Autodesk Inventor part; units mm, degrees
ref_plane "YZ Plane" through (0, 0, 0) normal (1, 0, 0) x (0, 1, 0)
ref_plane "XZ Plane" through (0, 0, 0) normal (0, 1, 0) x (-1, 0, 0)
ref_plane "XY Plane" through (0, 0, 0) normal (0, 0, 1) x (1, 0, 0)
sketch "Sketch1" plane through (0, 0, 0) normal (0, 0, 1) x (1, 0, 0)
  line L0 (0, 0) -> (-38.1, 0)
  line L1 (0, 0) -> (0, 114.3)
  line L2 (0, 114.3) -> (-38.1, 114.3)
  line L3 (-38.1, 114.3) -> (-38.1, 0)
  line L4 (-38.1, 114.3) -> (-31.75, 114.3)
  line L5 (-31.75, 114.3) -> (-31.75, 12.7)
  line L6 (0, 114.3) -> (-6.35, 114.3)
  line L7 (-6.35, 114.3) -> (-6.35, 12.7)
  circle A0 centre (-31.75, 12.7) radius 2.1463
  circle A1 centre (-6.35, 12.7) radius 2.1463
  dimension "d0" = 38.1
  dimension "d1" = 114.3
  dimension "d2" = 6.35
  dimension "d3" = 101.6
  dimension "d4" = 6.35
  dimension "d5" = 4.2926
  dimension "d6" = 4.2926
  dimension "d7" = 101.6
extrude "Plate1" add sketch "Sketch1" along normal blind 3.175
sketch "Sketch3" plane through (0, 0, 3.175) normal (0, 0, 1) x (1, 0, 0)
  line L0 (0, 114.3) -> (0, 0)
  line L1 (-38.1, 114.3) -> (0, 114.3)
  line L2 (-38.1, 0) -> (-38.1, 114.3)
  line L3 (-38.1, 114.3) -> (-38.1, 107.95)
  line L4 (-38.1, 107.95) -> (-31.75, 107.95)
  circle A0 centre (-31.75, 107.95) radius 3.3782
  line L5 (0, 114.3) -> (0, 107.95)
  line L6 (0, 107.95) -> (-6.35, 107.95)
  circle A1 centre (-6.35, 107.95) radius 3.3782
  line L7 (-38.1, 107.95) -> (-38.1, 57.15)
  line L8 (-38.1, 57.15) -> (-31.75, 57.15)
  line L9 (0, 57.15) -> (-6.35, 57.15)
  circle A2 centre (-31.75, 57.15) radius 3.3782
  circle A3 centre (-6.35, 57.15) radius 3.3782
  line L10 (-38.1, 114.3) -> (-38.1, 82.55)
  line L11 (-38.1, 82.55) -> (-19.05, 82.55)
  circle A4 centre (-19.05, 82.55) radius 14.2875
  dimension "d19" = 6.35
  dimension "d20" = 6.35
  dimension "d21" = 6.7564
  dimension "d22" = 6.35
  dimension "d23" = 6.35
  dimension "d24" = 6.7564
  dimension "d25" = 50.8
  dimension "d26" = 6.35
  dimension "d27" = 6.35
  dimension "d28" = 57.15
  dimension "d29" = 6.7564
  dimension "d30" = 6.7564
  dimension "d31" = 31.75
  dimension "d32" = 28.575
extrude "Cut1" cut sketch "Sketch3" against normal blind 3.175
equation "\"d33\" = Thickness"
equation "\"BendRadius\" = Thickness"
equation "\"BendReliefWidth\" = Thickness"
equation "\"BendReliefDepth\" = 0.5 * Thickness"
equation "\"CornerReliefSize\" = 4 * Thickness"
equation "\"MinimumRemnant\" = 2 * Thickness"
equation "\"TransitionRadius\" = BendRadius"
equation "\"JacobiRadiusSize\" = BendRadius"
equation "\"GapSize\" = Thickness"
equation "\"d8\" = BendRadius"
properties part number "upper pulley mount"
Work out the finished part from the listing and answer in its coordinate system (mm). Round coordinates to 2 decimals unless told otherwise and drop trailing zeros. Order: outer loops, then holes, each group sorted by start corner. A loop starts at its lowest first (then second) coordinate and runs counter-clockwise, first axis right, second up.
Q1. A cutting plane is placed at C-C, the plane z = 1.7. Count the separate pieces of the cut face and the enclosed holes in it, then the cut area to 3 significant figures.
Solution:
separate pieces: 1
enclosed holes: 7
area: 3,540 mm2
Q2. A cutting plane is placed at B-B, the plane x = -19.05. Determine the outline of the cut face in (y, z) (1 decimal).
Solution:
outline: (0, 0) - (68.3, 0) - (68.3, 3.2) - (0, 3.2) - close; (96.8, 0) - (114.3, 0) - (114.3, 3.2) - (96.8, 3.2) - close
Q3. The mould has two halves that part along X. Classify faces 1 (the flat face through (-38.1, 58, 2)), 2 (the flat face through (-19, 114.3, 2)), 3 (the cylindrical face through (-29.934, 59.999, 1.61)), 4 (the cylindrical face through (-6.8, 111.3, 1.6)): pulls with the +X half, pulls with the -X half, needs draft (parallel to the pull), parting line crosses it, or undercut.
Solution:
face 1: pulls with the -X half
face 2: needs draft
face 3: undercut
face 4: undercut
Q4. A cutting plane is placed at A-A, the plane y = 107.95. Determine the outline of the cut face in (x, z) (3 decimals).
Solution:
outline: (-38.1, 0) - (-35.128, 0) - (-35.128, 3.175) - (-38.1, 3.175) - close; (-28.372, 0) - (-9.728, 0) - (-9.728, 3.175) - (-28.372, 3.175) - close; (-2.972, 0) - (0, 0) - (0, 3.175) - (-2.972, 3.175) - close
Q5. Find the intervals of material crossed by line 1 along X through (y, z) = (12.7, 1.9); line 2 along Y through (x, z) = (-7, 0.95); line 3 along Y through (x, z) = (-6.35, 1.3), in increasing order.
Solution:
line 1: x = -38.1 to -33.9, -29.6 to -8.5, -4.2 to 0
line 2: y = 0 to 10.65, 14.75 to 53.83, 60.47 to 74.87, 90.23 to 104.63, 111.27 to 114.3
line 3: y = 0 to 10.55, 14.85 to 53.77, 60.53 to 76, 89.1 to 104.57, 111.33 to 114.3
Q6. Given pin 1 Ø4 at (x, y) = (-6.35, 12.7) entering from -Z, flat-ended and moving along its own axis, determine where the tip first touches the part or whether it passes through.
Solution:
pin 1: passes through
Q7. A cutting plane is placed at D-D, the plane y = 82.55. Determine the outline of the cut face in (x, z) (1 decimal), then the cut area to 3 significant figures.
Solution:
outline: (-38.1, 0) - (-33.3, 0) - (-33.3, 3.2) - (-38.1, 3.2) - close; (-4.8, 0) - (0, 0) - (0, 3.2) - (-4.8, 3.2) - close
area: 30.2 mm2
